Check sheet for the modelled part. Datum: model origin and axes. Units: mm. A direction names the side the tool comes from. Give positions to 0.01 mm unless a question says otherwise; leave off trailing zeros. Order: outer loops, then holes, each group sorted by start corner. A loop starts at its lowest first (then second) coordinate and runs counter-clockwise, first axis right, second up.
from build123d import *

# Parameters (mm, degrees)
SKETCH1_W                 = 57
SKETCH1_H                 = 33
BOSS_EXTRUDE1_DEPTH       = 14
SKETCH3_R                 = 3.35
CUT_EXTRUDE1_DEPTH        = 15
SKETCH4_R                 = 3.35
CUT_EXTRUDE2_DEPTH        = 15
SKETCH10_R                = 3.35
CUT_EXTRUDE5_DEPTH        = 15
SKETCH12_R                = 3.35
CUT_EXTRUDE6_DEPTH        = 15
F_8_32_TAPPED_HOLE1_D     = 3.4544
F_8_32_TAPPED_HOLE1_DEPTH = 5
F_8_32_TAPPED_HOLE1_TIP   = 1.037806461
F_0_535_40_TAPPED_HOLE1_D = 12.7


with BuildPart() as part:
    # Sketch1 → Boss-Extrude1 (new body)
    with BuildSketch(Plane(origin=(0, 0, 0), x_dir=(1, 0, 0), z_dir=(0, 1, 0))):
        with Locations((28.5, 16.5)):
            Rectangle(SKETCH1_W, SKETCH1_H)
    extrude(amount=BOSS_EXTRUDE1_DEPTH)

    # Sketch3 → Cut-Extrude1 (cut, through all)
    with BuildSketch(Plane.XZ):
        with Locations((6, -6.5)):
            Circle(SKETCH3_R)
    extrude(amount=-CUT_EXTRUDE1_DEPTH, mode=Mode.SUBTRACT)

    # Sketch4 → Cut-Extrude2 (cut, through all)
    with BuildSketch(Plane.XZ):
        with Locations((51, -26.5)):
            Circle(SKETCH4_R)
    extrude(amount=-CUT_EXTRUDE2_DEPTH, mode=Mode.SUBTRACT)

    # Sketch10 → Cut-Extrude5 (cut, through all)
    with BuildSketch(Plane.XZ):
        with Locations((6, -26.5)):
            Circle(SKETCH10_R)
    extrude(amount=-CUT_EXTRUDE5_DEPTH, mode=Mode.SUBTRACT)

    # Sketch12 → Cut-Extrude6 (cut, through all)
    with BuildSketch(Plane.XZ):
        with Locations((51, -6.5)):
            Circle(SKETCH12_R)
    extrude(amount=-CUT_EXTRUDE6_DEPTH, mode=Mode.SUBTRACT)

    # #8-32 Tapped Hole1
    with Locations(Plane(origin=(0, 0, -33), x_dir=(-1, 0, 0), z_dir=(0, 0, -1))):
        with Locations((-28.5, 7)):
            Hole(F_8_32_TAPPED_HOLE1_D / 2, depth=F_8_32_TAPPED_HOLE1_DEPTH)
            with Locations((0, 0, -(F_8_32_TAPPED_HOLE1_DEPTH + F_8_32_TAPPED_HOLE1_TIP / 2))):  # 118° drill point
                Cone(0, F_8_32_TAPPED_HOLE1_D / 2, F_8_32_TAPPED_HOLE1_TIP, mode=Mode.SUBTRACT)

    # 0.535-40 Tapped Hole1 (through all)
    with Locations(Plane(origin=(0, 14, 0), x_dir=(1, 0, 0), z_dir=(0, 1, 0))):
        with Locations((28.5, 16.5)):
            Hole(F_0_535_40_TAPPED_HOLE1_D / 2)


solid = part.part
1) Section check B-B, the plane z = -16.5. Record the cut outline in (x, y), then the cut area to 3 significant figures.
Recorded:
outline: (0, 0) - (22.15, 0) - (22.15, 14) - (0, 14) - close; (34.85, 0) - (57, 0) - (57, 14) - (34.85, 14) - close
area: 620 mm2
2) Section check D-D, the plane x = 25. Record the cut outline in (y, z).
Recorded:
outline: (0, -33) - (14, -33) - (14, -21.8) - (0, -21.8) - close; (0, -11.2) - (14, -11.2) - (14, 0) - (0, 0) - close
3) Depth check by flat-ended pin: pin 1 Ø6 at (x, z) = (51, -26.5) entering from +Y. Enter the tip coordinate at first touch or a pass-through.
Recorded:
pin 1: passes through
4) Set-up check for faces 4 (the face through (22, 0, -17)), 5 (the face through (29.429, 8.456, -30.465)): record each of +Z, -Z, +X, -X, +Y, -Y from which the full face is reachable in a straight line by a thin tool's end or side.
Recorded:
face 4: +Z, -Z, +X, -X, -Y
face 5: -Z
5) Draft check along Y on faces 1 (the face through (0, 7, -16)), 2 (the face through (28.223, 6.885, -27.142)), 3 (the face through (22, 14, -17)). Enter one of: +Y half, -Y half, draft (parallel to the pull), parting line (faces both ways), or undercut.
Recorded:
face 1: draft
face 2: undercut
face 3: +Y half
6) Section check A-A, the plane x = 51. Record the cut outline in (y, z), then the cut area to 3 significant figures.
Recorded:
outline: (0, -33) - (14, -33) - (14, -29.85) - (0, -29.85) - close; (0, -23.15) - (14, -23.15) - (14, -9.85) - (0, -9.85) - close; (0, -3.15) - (14, -3.15) - (14, 0) - (0, 0) - close
area: 274 mm2
7) Section check C-C, the plane y = 1.5. Record the cut outline in (x, z), then the cut area to 3 significant figures.
Recorded:
outline: (0, -33) - (57, -33) - (57, 0) - (0, 0) - close; hole circle Ø6.7 at (6, -26.5); hole circle Ø6.7 at (6, -6.5); hole circle Ø12.7 at (28.5, -16.5); hole circle Ø6.7 at (51, -26.5); hole circle Ø6.7 at (51, -6.5)
area: 1,610 mm2
8) Material ranges on L1, parallel to Z at x = 6, y = 5; L2, parallel to X at y = 7, z = -30.25; L3, parallel to X at y = 12, z = -25, recorded low to high.
Recorded:
L1: z = -33 to -29.85, -23.15 to -9.85, -3.15 to 0
L2: x = 0 to 26.77, 30.23 to 57
L3: x = 0 to 3, 9 to 48, 54 to 57
